Could you check a few things on this model? Use its own coordinates, in mm. A direction names the side the tool comes from. Round coordinates to 2 decimals unless told otherwise and drop trailing zeros. Write each loop counter-clockwise with the first axis right and the second up, starting at its lowest first coordinate (ties: lowest second). Pieces come first, ordered by that corner, then holes. Notation, with made-up numbers: (66, -27) -> (112, -27) arc R7 cw to (112, -14) -> close; hole circle Ø5 at (55, 32). An arc over 180 degrees is marked (long way). Answer in a Markdown table with one row per item. Add a question column.
```python
from build123d import *
from OCP.BRepFilletAPI import BRepFilletAPI_MakeChamfer

# Parameters (mm, degrees)
SKETCH_1_W          = 32.5
SKETCH_1_H          = 32
SKETCH_1_R          = 1
SKETCH_1_W_2        = 22.5
SKETCH_1_H_2        = 24.25
EXTRUDE_1_DEPTH     = 2
SKETCH_2_W          = 12
SKETCH_2_H          = 12
SKETCH_2_R          = 4
EXTRUDE_2_DEPTH     = 2.2
EXTRUDE_3_DEPTH     = 12
EXTRUDE_4_DEPTH     = 12
SKETCH_5_W          = 32.5
SKETCH_5_H          = 2
EXTRUDE_5_DEPTH     = 14
SKETCH_7_W          = 2
SKETCH_7_H          = 32
EXTRUDE_6_DEPTH     = 16
SKETCH_9_R          = 3.625
CUT_EXTRUDE_1_DEPTH = 1
SKETCH_10_R         = 2.25
CUT_EXTRUDE_2_DEPTH = 1
EXTRUDE_START       = -2
SKETCH_11_R         = 5
SKETCH_11_R_2       = 3.625
EXTRUDE_7_DEPTH     = 2
FILLET_1_R          = 1
SKETCH_12_R         = 3
SKETCH_12_R_2       = 1.5
EXTRUDE_8_DEPTH     = 2
FILLET_2_R          = 1
CUT_EXTRUDE_START   = 2
SKETCH_13_R         = 1.5
CUT_EXTRUDE_3_DEPTH = 2
SKETCH_19_W         = 3.200973594
SKETCH_19_H         = 7
CUT_EXTRUDE_7_DEPTH = 10
CUT_EXTRUDE_8_DEPTH = 42
SKETCH_22_R         = 0.75
CUT_EXTRUDE_9_DEPTH = 5
CHAMFER_1_SIZE      = 1
CHAMFER_1_SIZE2     = 2


with BuildPart() as part:
    # Sketch 1 → Extrude 1 (new body)
    with BuildSketch(Plane.XY):
        with Locations((-5.25, -6.125)):
            Rectangle(SKETCH_1_W, SKETCH_1_H)
        with Locations((-19, 0)):
            Circle(SKETCH_1_R, mode=Mode.SUBTRACT)
        with Locations(Location((8.5, 0, 0), (0, 0, 180))):
            Circle(SKETCH_1_R, mode=Mode.SUBTRACT)
        with Locations(Location((-19, -12.25, 0), (0, 0, 180))):
            Circle(SKETCH_1_R, mode=Mode.SUBTRACT)
        with Locations((8.5, -12.25)):
            Circle(SKETCH_1_R, mode=Mode.SUBTRACT)
        with Locations((-5.25, -6.125)):
            Rectangle(SKETCH_1_W_2, SKETCH_1_H_2, mode=Mode.SUBTRACT)
    extrude(amount=EXTRUDE_1_DEPTH)



with BuildPart() as body_2:
    # Sketch 2 → Extrude 2 (new body)
    with BuildSketch(Plane.XY.offset(9)):
        with Locations((-10.5, -12.25)):
            Rectangle(SKETCH_2_W, SKETCH_2_H)
        with Locations((-10.5, -12.25)):
            Circle(SKETCH_2_R, mode=Mode.SUBTRACT)
    extrude(amount=-EXTRUDE_2_DEPTH)


with BuildPart() as part_1:
    add(part.part)

    add(body_2.part)  # Extrude 3 merges body 2
    # Sketch 3 → Extrude 3 (add)
    with BuildSketch(Plane.ZY.offset(16.5)):
        Polygon((9, -18.25), (2, -18.25), (2, -22.125), (9, -20.25), align=None)
    extrude(amount=-EXTRUDE_3_DEPTH)

    # Sketch 4 → Extrude 4 (add)
    with BuildSketch(Plane.ZY.offset(16.5)):
        Polygon((6.8, -6.25), (9, -6.25), (9, 9.5), (2, 9.5), (2, 6), (6.8, 6), align=None)
    extrude(amount=-EXTRUDE_4_DEPTH)

    # Sketch 5 → Extrude 5 (add)
    with BuildSketch(Plane(origin=(0, 0, 0), x_dir=(-1, 0, 0), z_dir=(0, 0, -1))):
        with Locations((5.25, 8.875)):
            Rectangle(SKETCH_5_W, SKETCH_5_H)
        with Locations((5.25, -21.125)):
            Rectangle(SKETCH_5_W, SKETCH_5_H)
    extrude(amount=EXTRUDE_5_DEPTH)

    # Sketch 7 → Extrude 6 (add)
    with BuildSketch(Plane.XY.offset(2)):
        with Locations((-22.5, -6.125)):
            Rectangle(SKETCH_7_W, SKETCH_7_H)
        with Locations((12, -6.125)):
            Rectangle(SKETCH_7_W, SKETCH_7_H)
    extrude(amount=-EXTRUDE_6_DEPTH)

    # Sketch 9 → Cut-Extrude 1 (cut)
    with BuildSketch(Plane(origin=(-23.5, 0, 0), x_dir=(0, 0, -1), z_dir=(1, 0, 0))):
        with Locations(Location((8, -12.25, 0), (0, 0, 90))):
            Circle(SKETCH_9_R)
    extrude(amount=CUT_EXTRUDE_1_DEPTH, mode=Mode.SUBTRACT)

    # Sketch 10 → Cut-Extrude 2 (cut)
    with BuildSketch(Plane.ZY.offset(22.5)):
        with Locations(Location((-8, -12.25, 0), (0, 0, 270))):
            Circle(SKETCH_10_R)
    extrude(amount=-CUT_EXTRUDE_2_DEPTH, mode=Mode.SUBTRACT)

    # Sketch 11 → Extrude 7 (add)
    with BuildSketch(Plane(origin=(-23.5, 0, 0), x_dir=(0, 0, -1), z_dir=(1, 0, 0)).offset(EXTRUDE_START)):
        with Locations(Location((8, -12.25, 0), (0, 0, 90))):
            Circle(SKETCH_11_R)
        with Locations(Location((8, -12.25, 0), (0, 0, 90))):
            Circle(SKETCH_11_R_2, mode=Mode.SUBTRACT)
    extrude(amount=EXTRUDE_7_DEPTH)

    # Fillet 1
    fillet_1_edges = [part_1.edges().sort_by_distance(p)[0] for p in [
        (-23.5, -17.25, -8),
    ]]
    fillet(fillet_1_edges, radius=FILLET_1_R - 0.0001)  # a hair under: the kernel refuses the full size

    # Sketch 12 → Extrude 8 (add)
    with BuildSketch(Plane.ZY.offset(-13)):
        with Locations(Location((-8, -12.25, 0), (0, 0, 270))):
            Circle(SKETCH_12_R)
        with Locations(Location((-8, -12.25, 0), (0, 0, 270))):
            Circle(SKETCH_12_R_2, mode=Mode.SUBTRACT)
    extrude(amount=-EXTRUDE_8_DEPTH)

    # Fillet 2
    fillet_2_edges = [part_1.edges().sort_by_distance(p)[0] for p in [
        (13, -9.25, -8),
    ]]
    fillet(fillet_2_edges, radius=FILLET_2_R)

    # Sketch 13 → Cut-Extrude 3 (cut)
    with BuildSketch(Plane.ZY.offset(-13).offset(CUT_EXTRUDE_START)):
        with Locations(Location((-8, -12.25, 0), (0, 0, 270))):
            Circle(SKETCH_13_R)
    extrude(amount=-CUT_EXTRUDE_3_DEPTH, mode=Mode.SUBTRACT)

    # Sketch 19 → Cut-Extrude 7 (cut)
    with BuildSketch(Plane(origin=(0, 9.5, 0), x_dir=(1, 0, 0), z_dir=(0, 1, 0))):
        with Locations((-10.5, -5.5)):
            Rectangle(SKETCH_19_W, SKETCH_19_H)
    extrude(amount=-CUT_EXTRUDE_7_DEPTH, mode=Mode.SUBTRACT)

    # Sketch 20 → Cut-Extrude 8 (cut)
    with BuildSketch(Plane(origin=(0, 9.875, 0), x_dir=(1, 0, 0), z_dir=(0, 1, 0))):
        with BuildLine():
            Line((-6.75, 10.5), (-6.75, 1.5))
            ThreePointArc((-6.75, 1.5), (-7.042893219, 0.792893219), (-7.75, 0.5))
            Line((-7.75, 0.5), (-8.75, 0.5))
            ThreePointArc((-8.75, 0.5), (-9.457106781, 0.792893219), (-9.75, 1.5))
            Line((-9.75, 1.5), (-9.75, 10.5))
            ThreePointArc((-9.75, 10.5), (-9.457106781, 11.207106781), (-8.75, 11.5))
            Line((-8.75, 11.5), (-7.75, 11.5))
            ThreePointArc((-7.75, 11.5), (-7.042893219, 11.207106781), (-6.75, 10.5))
        make_face()
        with BuildLine():
            Line((8.25, 10.5), (8.25, 1.5))
            ThreePointArc((8.25, 1.5), (8.542893219, 0.792893219), (9.25, 0.5))
            Line((9.25, 0.5), (10.25, 0.5))
            ThreePointArc((10.25, 0.5), (10.957106781, 0.792893219), (11.25, 1.5))
            Line((11.25, 1.5), (11.25, 10.5))
            ThreePointArc((11.25, 10.5), (10.957106781, 11.207106781), (10.25, 11.5))
            Line((10.25, 11.5), (9.25, 11.5))
            ThreePointArc((9.25, 11.5), (8.542893219, 11.207106781), (8.25, 10.5))
        make_face()
        with BuildLine():
            Line((-14.75, 11.5), (-13.75, 11.5))
            ThreePointArc((-13.75, 11.5), (-13.042893219, 11.207106781), (-12.75, 10.5))
            Line((-12.75, 10.5), (-12.75, 1.5))
            ThreePointArc((-12.75, 1.5), (-13.042893219, 0.792893219), (-13.75, 0.5))
            Line((-13.75, 0.5), (-14.75, 0.5))
            ThreePointArc((-14.75, 0.5), (-15.457106781, 0.792893219), (-15.75, 1.5))
            Line((-15.75, 1.5), (-15.75, 10.5))
            ThreePointArc((-15.75, 10.5), (-15.457106781, 11.207106781), (-14.75, 11.5))
        make_face()
        with BuildLine():
            Line((-20.75, 11.5), (-19.75, 11.5))
            ThreePointArc((-19.75, 11.5), (-19.042893219, 11.207106781), (-18.75, 10.5))
            Line((-18.75, 10.5), (-18.75, 1.5))
            ThreePointArc((-18.75, 1.5), (-19.042893219, 0.792893219), (-19.75, 0.5))
            Line((-19.75, 0.5), (-20.75, 0.5))
            ThreePointArc((-20.75, 0.5), (-21.457106781, 0.792893219), (-21.75, 1.5))
            Line((-21.75, 1.5), (-21.75, 10.5))
            ThreePointArc((-21.75, 10.5), (-21.457106781, 11.207106781), (-20.75, 11.5))
        make_face()
        with BuildLine():
            Line((2.25, 10.5), (2.25, 1.5))
            ThreePointArc((2.25, 1.5), (2.542893219, 0.792893219), (3.25, 0.5))
            Line((3.25, 0.5), (4.25, 0.5))
            ThreePointArc((4.25, 0.5), (4.957106781, 0.792893219), (5.25, 1.5))
            Line((5.25, 1.5), (5.25, 10.5))
            ThreePointArc((5.25, 10.5), (4.957106781, 11.207106781), (4.25, 11.5))
            Line((4.25, 11.5), (3.25, 11.5))
            ThreePointArc((3.25, 11.5), (2.542893219, 11.207106781), (2.25, 10.5))
        make_face()
        with BuildLine():
            Line((-1.75, 11.5), (-2.75, 11.5))
            ThreePointArc((-2.75, 11.5), (-3.457106781, 11.207106781), (-3.75, 10.5))
            Line((-3.75, 10.5), (-3.75, 1.5))
            ThreePointArc((-3.75, 1.5), (-3.457106781, 0.792893219), (-2.75, 0.5))
            Line((-2.75, 0.5), (-1.75, 0.5))
            ThreePointArc((-1.75, 0.5), (-1.042893219, 0.792893219), (-0.75, 1.5))
            Line((-0.75, 1.5), (-0.75, 10.5))
            ThreePointArc((-0.75, 10.5), (-1.042893219, 11.207106781), (-1.75, 11.5))
        make_face()
    extrude(amount=-CUT_EXTRUDE_8_DEPTH, mode=Mode.SUBTRACT)

    # Sketch 22 → Cut-Extrude 9 (cut)
    with BuildSketch(Plane(origin=(0, 9.5, 0), x_dir=(1, 0, 0), z_dir=(0, 1, 0))):
        with Locations(Location((-6.7, -4.8, 0), (0, 0, 270))):
            Circle(SKETCH_22_R)
        with Locations((-14.3, -4.8)):
            Circle(SKETCH_22_R)
    extrude(amount=-CUT_EXTRUDE_9_DEPTH, mode=Mode.SUBTRACT)

    # Chamfer 1: one chamfer whose edges measure the first distance from different faces: ONE call of the kernel's chamfer builder (chamfer() names one face for all edges)
    chamfer_1_edges_1 = [part_1.edges().sort_by_distance(p)[0] for p in [
        (-14.300243398, 9.5, 9),
    ]]
    chamfer_1_side_1 = [part_1.faces().sort_by_distance(p)[0] for p in [
        (-16.417322484, 9.5, 5.5),
    ]]
    chamfer_1_edges_2 = [part_1.edges().sort_by_distance(p)[0] for p in [
        (-6.699756602, 9.5, 9),
    ]]
    chamfer_1_side_2 = [part_1.faces().sort_by_distance(p)[0] for p in [
        (-8.816835687, 9.5, 5.5),
    ]]
    chamfer_1 = BRepFilletAPI_MakeChamfer(part_1.part.solid().wrapped)
    for e in chamfer_1_edges_1:
        chamfer_1.Add(CHAMFER_1_SIZE, CHAMFER_1_SIZE2, e.wrapped, chamfer_1_side_1[0].wrapped)  # the first distance lies on this face
    for e in chamfer_1_edges_2:
        chamfer_1.Add(CHAMFER_1_SIZE, CHAMFER_1_SIZE2, e.wrapped, chamfer_1_side_2[0].wrapped)  # the first distance lies on this face
    add(Compound.cast(chamfer_1.Shape()), mode=Mode.REPLACE)


solid = part_1.part
```
(1) Suppose I cut it at B-B, the plane y = 6.5. Please give me the cut outline in (x, z).
(2) For P1, Ø5, axis at y = 3, z = -6, coming from the +X side; P2, Ø2, axis at y = 9, z = -7, coming from the -X side; P3, Ø0.8, axis at x = 3.5, y = 8.5, coming from the +Z side, each with a flat end and sliding along its axis, tell me the tip position at first contact or that it passes through.
(3) Suppose I cut it at D-D, the plane y = -5. Please give me the cut outline in (x, z).
(4) I need wall thicknesses on L1, parallel to X at y = 8.75, z = 4.8; L2, parallel to Y at x = -19, z = 1.55 (3 decimals); L3, parallel to Z at x = -22.1, y = -12.25. Which ranges of each line are inside material? Lowest first, please.
(5) If we mould it in two halves opening along X, with no side actions, what happens to faces 4 (the face through (-6, 9.875, -6)), 5 (the face through (-16.5, -6, 7)), 6 (the face through (-8, -21, -11.5)), 7 (the face through (-3.449, 8.889, -11.215))? For each: pulls with the +X half, pulls with the -X half, needs draft (parallel to the pull), parting line crosses it, or undercut.
(6) Suppose I cut it at A-A, the plane x = -10.5. Please give me the cut outline in (y, z) (3 decimals), then the cut area to 3 significant figures.
(7) On a 3-axis mill with a long thin cutter (end or side, diameter ignored), from which of +Z, -Z, +X, -X, +Y, -Y can I reach the whole of each face in a straight line? I mean faces 1 (the face through (9.3, 0.6, 1)), 2 (the face through (-21.75, -6, -6)), 3 (the face through (-11, -6, 6.8)). Say none if no direction works.
(8) Suppose I cut it at C-C, the plane z = 1. Please give me the cut outline in (x, y) (3 decimals), then the cut area to 3 significant figures.
Response:
| question | item | result |
|---|---|---|
| 1 | outline | (-23.5, -14) -> (-21.5, -14) -> (-21.5, -11.16) arc R1 cw to (-21.75, -10.5) -> (-21.75, -1.5) arc R1 cw to (-21.5, -0.84) -> (-21.5, 0) -> (11, 0) -> (11, -0.84) arc R1 cw to (11.25, -1.5) -> (11.25, -10.5) arc R1 cw to (11, -11.16) -> (11, -14) -> (13, -14) -> (13, 2) -> (-4.5, 2) -> (-4.5, 9) -> (-8.9, 9) -> (-8.9, 2) -> (-12.1, 2) -> (-12.1, 9) -> (-16.5, 9) -> (-16.5, 2) -> (-23.5, 2) -> close; hole circle Ø1.5 at (-14.3, 4.8); hole circle Ø1.5 at (-6.7, 4.8) |
| 2 | P1 | x = 13 |
| 2 | P2 | x = -23.5 |
| 2 | P3 | z = 2 |
| 3 | outline | (-23.5, -14) -> (-21.5, -14) -> (-21.5, -11.16) arc R1 cw to (-21.75, -10.5) -> (-21.75, -1.5) arc R1 cw to (-21.5, -0.84) -> (-21.5, 0) -> (-16.5, 0) -> (-16.5, 2) -> (-23.5, 2) -> close; (-16.5, 6.8) -> (-4.5, 6.8) -> (-4.5, 9) -> (-16.5, 9) -> close; (6, 0) -> (11, 0) -> (11, -0.84) arc R1 cw to (11.25, -1.5) -> (11.25, -10.5) arc R1 cw to (11, -11.16) -> (11, -14) -> (13, -14) -> (13, 2) -> (6, 2) -> close |
| 4 | L1 | -16.5 to -15.05, -13.55 to -12.1, -8.9 to -7.45, -5.95 to -4.5 |
| 4 | L2 | -22.125 to -13.25, -11.25 to -1, 1 to 9.875 |
| 4 | L3 | -14 to -10.25, -5.75 to 2 |
| 5 | face 4 | needs draft |
| 5 | face 5 | pulls with the -X half |
| 5 | face 6 | undercut |
| 5 | face 7 | undercut |
| 6 | outline | (-22.125, -14) -> (-20.125, -14) -> (-20.125, 0) -> (-18.25, 0) -> (-18.25, 6.8) -> (-16.25, 6.8) -> (-16.25, 9) -> (-20.25, 9) -> (-22.125, 2) -> close; (-8.25, 6.8) -> (-0.5, 6.8) -> (-0.5, 9) -> (-8.25, 9) -> close; (6, 0) -> (7.875, 0) -> (7.875, -14) -> (9.875, -14) -> (9.875, 2) -> (6, 2) -> close |
| 6 | area | 114 mm² |
| 7 | face 1 | +Z, -Z |
| 7 | face 2 | +Y, -Y |
| 7 | face 3 | -Z, +X, -X |
| 8 | outline | (-23.5, -22.125) -> (13, -22.125) -> (13, 9.875) -> (-23.5, 9.875) -> close; hole circle Ø2 at (-19, -12.25); hole circle Ø2 at (-19, 0); hole (-16.5, -18.25) -> (6, -18.25) -> (6, 6) -> (-16.5, 6) -> close; hole circle Ø2 at (8.5, -12.25); hole circle Ø2 at (8.5, 0) |
| 8 | area | 610 mm² |
